Could you check a few things on this model? Use its own coordinates, in mm. Face numbers are marked on the shaded views. Give positions to 0.01 mm unless a question says otherwise; leave off trailing zeros. Loops run counter-clockwise (first coordinate to the right, second up) from the corner with the lowest first, then second, coordinate; pieces in that order, holes last. Notation, with made-up numbers: M 54.25,9.5 L 97.25,9.5 A28 ccw 97.25,46.5 Z; hole C 79.25,-39 d11. An arc over 180 degrees is marked long. Use CSV: the item, a comma, the result in double quotes.
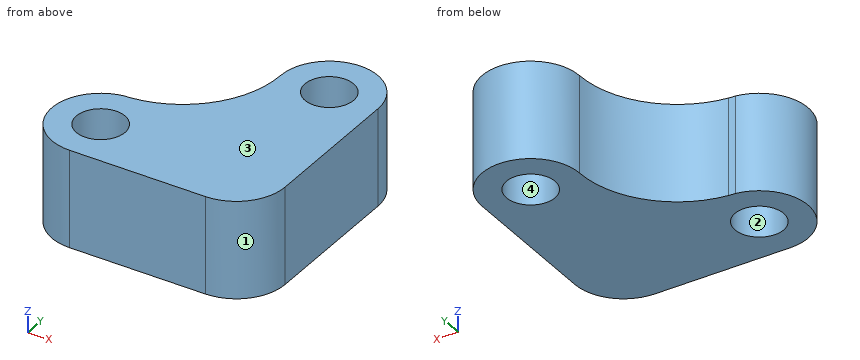
```python
from build123d import *

# Parameters (mm, degrees)
F0_R     = 2.5
F1_DEPTH = 10


with BuildPart() as f1:
    # F0 (on Top) → F1 (new body)
    with BuildSketch(Plane.XY):
        with BuildLine():
            ThreePointArc((0, -5), (-3.5355339059, 3.5355339059), (5, 0))
            Line((5, 0), (5, 15))
            ThreePointArc((5, 15), (0, 10), (-5, 15))
            ThreePointArc((-5, 15), (-7.5406677948, 8.2821226215), (-13.9291371274, 5))
            ThreePointArc((-13.9291371274, 5), (-10.3936032215, 3.5355339059), (-8.9291371274, 0))
            ThreePointArc((-8.9291371274, 0), (-10.3936032215, -3.5355339059), (-13.9291371274, -5))
            Line((-13.9291371274, -5), (0, -5))
        make_face()
        with BuildLine():
            ThreePointArc((-14.6420213859, 4.9489186732), (-18.9163504458, -0.3573560088), (-13.9291371274, -5))
            ThreePointArc((-13.9291371274, -5), (-10.3936032215, -3.5355339059), (-8.9291371274, 0))
            ThreePointArc((-8.9291371274, 0), (-10.3936032215, 3.5355339059), (-13.9291371274, 5))
            ThreePointArc((-13.9291371274, 5), (-14.2851227554, 4.9680884652), (-14.6420213859, 4.9489186732))
        make_face()
        with Locations((-13.9291371274, 0)):
            Circle(F0_R, mode=Mode.SUBTRACT)
        with BuildLine():
            ThreePointArc((0, -5), (3.5355339059, -3.5355339059), (5, 0))
            ThreePointArc((5, 0), (-3.5355339059, 3.5355339059), (0, -5))
        make_face()
        with BuildLine():
            ThreePointArc((5, 15), (0, 20), (-5, 15))
            ThreePointArc((-5, 15), (0, 10), (5, 15))
        make_face()
        with Locations((0, 15)):
            Circle(F0_R, mode=Mode.SUBTRACT)
    extrude(amount=F1_DEPTH)


solid = f1.part
```
1. Please list where these lines run through material, in increasing order: line 1 (Y direction, x = 0, z = 7.25); line 2 (Y direction, x = 2, z = 9.25); line 3 (X direction, y = 12.75, z = 6).
Outcome:
line 1,"-5 to 12.5, 17.5 to 20"
line 2,"-4.58 to 13.5, 16.5 to 19.58"
line 3,"-5.24 to -1.09, 1.09 to 5"
2. I want a section at B-B, the plane z = 3. List the corners of the cut face in (x, y) for me, then the cut area to 3 significant figures.
Outcome:
outline,"M -14.64,4.95 A5 ccw -13.93,-5 L 0,-5 A5 ccw 5,0 L 5,15 A5 ccw long -5,14.96 A10 cw Z; hole C -13.93,0 d5; hole C 0,15 d5"
area,"344 mm2"
3. I want a section at A-A, the plane y = -1.5. List the corners of the cut face in (x, z) for me, then the cut area to 3 significant figures.
Outcome:
outline,"M -18.7,0 L -15.93,0 L -15.93,10 L -18.7,10 Z; M -11.93,0 L 4.77,0 L 4.77,10 L -11.93,10 Z"
area,"195 mm2"
4. I want a section at C-C, the plane x = -9.5. List the corners of the cut face in (y, z) for me, then the cut area to 3 significant figures.
Outcome:
outline,"M -5,0 L 6.59,0 L 6.59,10 L -5,10 Z"
area,"116 mm2"
5. I'm going to push flat-ended pins straight in: pin 1 Ø4 at (y, z) = (12.5, 6) entering from -X; pin 2 Ø1.5 at (y, z) = (15, 8.5) entering from -X; pin 3 Ø4 at (y, z) = (17.5, 2) entering from +X. Where does each tip first touch, or does it pass through?
Outcome:
pin 1,"x = -6.04"
pin 2,"x = -5.02"
pin 3,"x = 4.97"
6. I want a section at D-D, the plane y = 6.25. List the corners of the cut face in (x, z) for me, then the cut area to 3 significant figures.
Outcome:
outline,"M -10.06,0 L 5,0 L 5,10 L -10.06,10 Z"
area,"151 mm2"
7. If we mould it in two halves opening along X, with no side actions, what happens to the marked faces 1, 2, 3 and 4? For each: +X half, -X half, draft (parallel to the pull), parting line (faces both ways), or undercut.
Outcome:
face 1,"+X half"
face 2,"undercut"
face 3,"draft"
face 4,"undercut"
